```python
from build123d import *

# Parameters (mm, degrees)
F0_W          = 22.5927522406
F0_H          = 49.5025906712
F1_DEPTH      = 10.16
F2_DEPTH      = 3.81
F3_W          = 11.2244246993
F3_H          = 99.0051813424
F4_DEPTH      = 25.4
F6_DEPTH      = 10.16
F7_R          = 2.54
F8_W          = 33.9610797819
F8_H          = 38.1342638284
F8_H_2        = 37.1269418392
F9_DEPTH      = 5.842
F10_R         = 2.54
F11_W         = 99.0051813424
F11_H         = 67.9221570026
F12_DEPTH     = 10.414
F13_W         = 38.620619569
F13_H         = 17.018
F13_W_2       = 37.6479080878
F14_DEPTH     = 3.302
F15_T1_DEPTH  = 88.9685276568
F15_T6_DEPTH  = 27.94
F15_T11_DEPTH = 27.94
F16_W         = 1.1473407503
F16_H         = 14.478
F17_DEPTH     = 3.302
F18_W         = 19.139082171
F18_H         = 29.1566260799
F18_W_2       = 6.5123029053
F18_H_2       = 0.8140355349
F18_W_3       = 18.2694643736
F18_W_4       = 7.5298482552
F18_W_5       = 18.2365168585
F18_W_6       = 7.1228295565
F18_W_7       = 18.1018151343
F18_W_8       = 7.1228314191
F19_DEPTH     = 0.254
F20_DEPTH     = 1.524


# Not quite as in the source:
# - a fillet or chamfer that OpenCascade refuses, or shapes differently, is made with other operations: its cross-section is extruded or revolved along the edge and cut away or added
# - a feature names something its author has since deleted; it is built from what else it names


with BuildPart() as f1:
    # F0 (on Top) → F1 (new body)
    with BuildSketch(Plane.XY):
        with BuildLine():
            Line((-35.3594812499, 51.6611337662), (-36.6952344775, 51.6611337662))
            Line((-36.6952344775, 51.6611337662), (-36.6952344775, 50.3253805386))
            ThreePointArc((-36.6952344775, 50.3253805386), (-36.1400711383, 51.105970427), (-35.3594812499, 51.6611337662))
        make_face()
        with BuildLine():
            ThreePointArc((-32.8504798068, 51.6611337662), (-34.1049805284, 51.9489325583), (-35.3594812499, 51.6611337662))
            Line((-35.3594812499, 51.6611337662), (-32.8504798068, 51.6611337662))
        make_face()
        with BuildLine():
            Line((-32.8504798068, 51.6611337662), (-35.3594812499, 51.6611337662))
            ThreePointArc((-35.3594812499, 51.6611337662), (-36.1400711383, 51.105970427), (-36.6952344775, 50.3253805386))
            Line((-36.6952344775, 50.3253805386), (-36.6952344775, 47.8163790954))
            ThreePointArc((-36.6952344775, 47.8163790954), (-33.4614356183, 46.2656993361), (-31.2269277871, 49.070879817))
            ThreePointArc((-31.2269277871, 49.070879817), (-31.6663634179, 50.5993869876), (-32.8504798068, 51.6611337662))
        make_face()
        with BuildLine():
            Line((-36.6952344775, 47.8163790954), (-36.6952344775, 50.3253805386))
            ThreePointArc((-36.6952344775, 50.3253805386), (-36.9830332696, 49.070879817), (-36.6952344775, 47.8163790954))
        make_face()
        with BuildLine():
            Line((-14.1024822369, 51.6611337662), (-32.8504798068, 51.6611337662))
            ThreePointArc((-32.8504798068, 51.6611337662), (-31.6663634179, 50.5993869876), (-31.2269277871, 49.070879817))
            ThreePointArc((-31.2269277871, 49.070879817), (-33.4614356183, 46.2656993361), (-36.6952344775, 47.8163790954))
            Line((-36.6952344775, 47.8163790954), (-36.6952344775, 2.158543095))
            Line((-36.6952344775, 2.158543095), (-14.1024822369, 2.158543095))
            Line((-14.1024822369, 2.158543095), (-14.1024822369, 51.6611337662))
        make_face()
        with Locations((-2.8061061166, 26.9098384306)):
            Rectangle(F0_W, F0_H)
        with BuildLine():
            Line((-14.1024822369, 2.158543095), (-36.6952344775, 2.158543095))
            Line((-36.6952344775, 2.158543095), (-36.6952344775, -43.4992929054))
            ThreePointArc((-36.6952344775, -43.4992929054), (-33.4614356183, -41.9486131461), (-31.2269277871, -44.753793627))
            ThreePointArc((-31.2269277871, -44.753793627), (-31.6663634179, -46.2823007976), (-32.8504798068, -47.3440475762))
            Line((-32.8504798068, -47.3440475762), (-14.1024822369, -47.3440475762))
            Line((-14.1024822369, -47.3440475762), (-14.1024822369, 2.158543095))
        make_face()
        with Locations((-2.8061061166, -22.5927522406)):
            Rectangle(F0_W, F0_H)
        with BuildLine():
            ThreePointArc((-31.2269277871, -44.753793627), (-33.4614356183, -41.9486131461), (-36.6952344775, -43.4992929054))
            Line((-36.6952344775, -43.4992929054), (-36.6952344775, -46.0082943486))
            ThreePointArc((-36.6952344775, -46.0082943486), (-36.1400711383, -46.788884237), (-35.3594812499, -47.3440475762))
            Line((-35.3594812499, -47.3440475762), (-32.8504798068, -47.3440475762))
            ThreePointArc((-32.8504798068, -47.3440475762), (-31.6663634179, -46.2823007976), (-31.2269277871, -44.753793627))
        make_face()
        with BuildLine():
            Line((-36.6952344775, -46.0082943486), (-36.6952344775, -43.4992929054))
            ThreePointArc((-36.6952344775, -43.4992929054), (-36.9830332696, -44.753793627), (-36.6952344775, -46.0082943486))
        make_face()
        with BuildLine():
            ThreePointArc((-35.3594812499, -47.3440475762), (-36.1400711383, -46.788884237), (-36.6952344775, -46.0082943486))
            Line((-36.6952344775, -46.0082943486), (-36.6952344775, -47.3440475762))
            Line((-36.6952344775, -47.3440475762), (-35.3594812499, -47.3440475762))
        make_face()
        with BuildLine():
            ThreePointArc((-35.3594812499, -47.3440475762), (-34.1049805284, -47.6318463683), (-32.8504798068, -47.3440475762))
            Line((-32.8504798068, -47.3440475762), (-35.3594812499, -47.3440475762))
        make_face()
    extrude(amount=F1_DEPTH)

    # F0 (on Top) → F2 (join)
    with BuildSketch(Plane.XY):
        with BuildLine():
            Line((-32.8504798068, 51.6611337662), (-35.3594812499, 51.6611337662))
            ThreePointArc((-35.3594812499, 51.6611337662), (-36.1400711383, 51.105970427), (-36.6952344775, 50.3253805386))
            Line((-36.6952344775, 50.3253805386), (-36.6952344775, 47.8163790954))
            ThreePointArc((-36.6952344775, 47.8163790954), (-33.4614356183, 46.2656993361), (-31.2269277871, 49.070879817))
            ThreePointArc((-31.2269277871, 49.070879817), (-31.6663634179, 50.5993869876), (-32.8504798068, 51.6611337662))
        make_face()
        with BuildLine():
            ThreePointArc((-31.2269277871, -44.753793627), (-33.4614356183, -41.9486131461), (-36.6952344775, -43.4992929054))
            Line((-36.6952344775, -43.4992929054), (-36.6952344775, -46.0082943486))
            ThreePointArc((-36.6952344775, -46.0082943486), (-36.1400711383, -46.788884237), (-35.3594812499, -47.3440475762))
            Line((-35.3594812499, -47.3440475762), (-32.8504798068, -47.3440475762))
            ThreePointArc((-32.8504798068, -47.3440475762), (-31.6663634179, -46.2823007976), (-31.2269277871, -44.753793627))
        make_face()
    extrude(amount=-F2_DEPTH)

    # F3 (on face) → F4 (join)
    with BuildSketch(Plane.XY.offset(10.16)):
        with Locations((2.878057654, 2.158543095)):
            Rectangle(F3_W, F3_H)
    extrude(amount=F4_DEPTH)

    # F5 (on face) → F6 (join)
    with BuildSketch(Plane.XY.offset(10.16)):
        Polygon((-2.7341546956, 40.4367111623), (-2.7341546956, 51.6611337662), (-32.8504798068, 51.6611337662), (-35.3594812499, 51.6611337662), (-36.6952344775, 51.6611337662), (-36.6952344775, 50.3253805386), (-36.6952344775, 47.8163790954), (-36.6952344775, 40.4367111623), align=None)
        Polygon((-2.7341546956, -47.3440475762), (-2.7341546956, -35.8318164945), (-36.6952344775, -35.8318164945), (-36.6952344775, -43.4992929054), (-36.6952344775, -46.0082943486), (-36.6952344775, -47.3440475762), (-35.3594812499, -47.3440475762), (-32.8504798068, -47.3440475762), align=None)
    extrude(amount=F6_DEPTH)

    # F7
    f7_edges = [f1.edges().sort_by_distance(p)[0] for p in [
        (-2.734155, 2.158543, 35.56),
        (-19.714695, -35.831816, 20.32),
        (-19.714695, -47.344048, 20.32),
        (-19.714695, 51.661134, 20.32),
        (-19.714695, 40.436711, 20.32),
    ]]
    fillet(f7_edges, radius=F7_R)

    # F8 (on face) → F9 (join)
    with BuildSketch(Plane.XY.offset(10.16)):
        with Locations((-19.7146945866, 21.3695792481)):
            Rectangle(F8_W, F8_H)
        with Locations((-19.7146945866, -17.2683455748)):
            Rectangle(F8_W, F8_H_2)
    extrude(amount=F9_DEPTH)

    # F10
    f10_edges = [f1.edges().sort_by_distance(p)[0] for p in [
        (-19.714695, 1.295125, 16.002),
        (-19.714695, 2.302447, 16.002),
        (-36.695234, -17.268346, 16.002),
        (-36.695234, 21.369579, 16.002),
    ]]
    fillet(f10_edges, radius=F10_R)

    # F11 (on face) → F12 (join)
    with BuildSketch(Plane.YZ.offset(8.4902700037)):
        with Locations((2.158543095, 30.0757006044)):
            Rectangle(F11_W, F11_H)
    extrude(amount=-F12_DEPTH)

    # F13 (on face) → F14 (join)
    with BuildSketch(Plane(origin=(-2.7341546956, 0, 0), x_dir=(0, -1, 0), z_dir=(-1, 0, 0))):
        with Locations((-21.1264013778, 24.511)):
            Rectangle(F13_W, F13_H)
        with Locations((17.0078624506, 24.511)):
            Rectangle(F13_W_2, F13_H)
    extrude(amount=F14_DEPTH)

    # F15: fillet of radius 2.54 on 3 edges, made by hand

    # F15_s2 → F15_t1 (cut)
    with BuildSketch(Plane.XZ.offset(-46.7867111623)):
        with BuildLine():
            ThreePointArc((-6.0361546956, 30.48), (-5.2922059199, 32.2760512242), (-3.4961546956, 33.02))
            Line((-3.4961546956, 33.02), (-6.0361546956, 33.02))
            Line((-6.0361546956, 33.02), (-6.0361546956, 30.48))
        make_face()
    extrude(amount=F15_T1_DEPTH, mode=Mode.SUBTRACT)


with BuildPart() as f15_tool4:
    # F15_s5 → F15_t6 (new body)
    with BuildSketch(Plane.XY.offset(39.37)):
        with BuildLine():
            ThreePointArc((-6.0361546956, 37.8967111623), (-5.2922059199, 39.6927623865), (-3.4961546956, 40.4367111623))
            Line((-3.4961546956, 40.4367111623), (-6.0361546956, 40.4367111623))
            Line((-6.0361546956, 40.4367111623), (-6.0361546956, 37.8967111623))
        make_face()
    extrude(amount=-F15_T6_DEPTH)

    split(bisect_by=Plane.XY.offset(16.002), keep=Keep.TOP)


with BuildPart() as f1_1:
    add(f1.part)

    # F15_t3: cut F15_tool4
    add(f15_tool4.part, mode=Mode.SUBTRACT)


with BuildPart() as f15_tool9:
    # F15_s10 → F15_t11 (new body)
    with BuildSketch(Plane.XY.offset(11.43)):
        with BuildLine():
            ThreePointArc((-6.0361546956, -33.2918164945), (-5.2922059199, -35.0878677187), (-3.4961546956, -35.8318164945))
            Line((-3.4961546956, -35.8318164945), (-6.0361546956, -35.8318164945))
            Line((-6.0361546956, -35.8318164945), (-6.0361546956, -33.2918164945))
        make_face()
    extrude(amount=F15_T11_DEPTH)

    split(bisect_by=Plane.XY.offset(16.002), keep=Keep.TOP)


with BuildPart() as f1_2:
    add(f1_1.part)

    # F15_t8: cut F15_tool9
    add(f15_tool9.part, mode=Mode.SUBTRACT)

    # F16 (on face) → F17 (cut)
    with BuildSketch(Plane(origin=(-6.0361546956, 0, 0), x_dir=(0, -1, 0), z_dir=(-1, 0, 0))):
        with Locations((-1.7287769588, 23.241)):
            Rectangle(F16_W, F16_H)
    extrude(amount=-F17_DEPTH, mode=Mode.SUBTRACT)

    # F18 (on face) → F19 (join)
    with BuildSketch(Plane(origin=(-1.9237299963, 0, 0), x_dir=(0, -1, 0), z_dir=(-1, 0, 0))):
        with Locations((-30.8671663515, 49.4584660657)):
            Rectangle(F18_W, F18_H)
        with Locations((-30.3225759417, 61.080571264)):
            Rectangle(F18_W_2, F18_H_2, mode=Mode.SUBTRACT)
        with Locations((-11.2932752818, 49.4584660657)):
            Rectangle(F18_W_3, F18_H)
        with Locations((-11.4979553036, 61.080571264)):
            Rectangle(F18_W_4, F18_H_2, mode=Mode.SUBTRACT)
        with Locations((7.7183801332, 49.4584660657)):
            Rectangle(F18_W_5, F18_H)
        with Locations((7.9371919855, 61.080571264)):
            Rectangle(F18_W_6, F18_H_2, mode=Mode.SUBTRACT)
        with Locations((26.7809126526, 49.4584660657)):
            Rectangle(F18_W_7, F18_H)
        with Locations((27.0670773461, 61.080571264)):
            Rectangle(F18_W_8, F18_H_2, mode=Mode.SUBTRACT)
    extrude(amount=F19_DEPTH)

    # F18 (on face) → F20 (join)
    with BuildSketch(Plane(origin=(-1.9237299963, 0, 0), x_dir=(0, -1, 0), z_dir=(-1, 0, 0))):
        with Locations((27.0670773461, 61.080571264)):
            Rectangle(F18_W_8, F18_H_2)
        with Locations((7.9371919855, 61.080571264)):
            Rectangle(F18_W_6, F18_H_2)
        with Locations((-11.4979553036, 61.080571264)):
            Rectangle(F18_W_4, F18_H_2)
        with Locations((-30.3225759417, 61.080571264)):
            Rectangle(F18_W_2, F18_H_2)
    extrude(amount=F20_DEPTH)


solid = f1_2.part
```
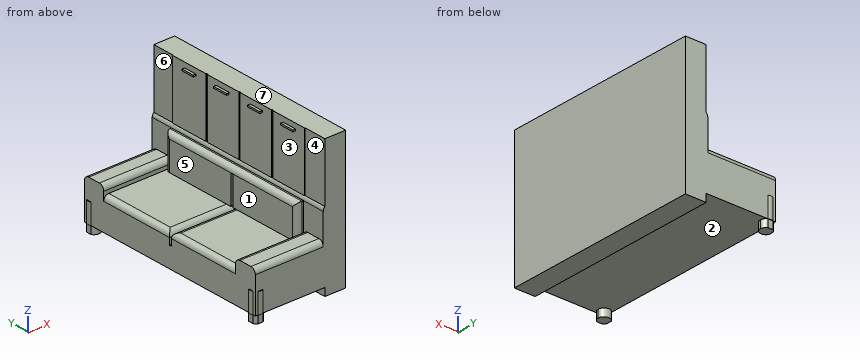
The model under review builds one solid part; all positions refer to its coordinate system, in mm. Face numbers are marked on the shaded views. A direction names the side the tool comes from. Round coordinates to 2 decimals unless told otherwise and drop trailing zeros. Order: outer loops, then holes, each group sorted by start corner. A loop starts at its lowest first (then second) coordinate and runs counter-clockwise, first axis right, second up. Notation, with made-up numbers: (68, -34) -> (82, -34) arc R23 ccw to (82, -22) -> close; hole circle Ø1 at (77.5, -27.5). An arc over 180 degrees is marked (long way). One line per item, written item: value. Start each with the question number.
Q1. Take a section at C-C (z = 22.5). Write out the cut boundary in (x, y).
Q2. Take a section at D-D (y = 35.5). Write out the cut boundary in (x, z), and give its area (3 significant figures).
Q3. Clearance check with flat-ended pins moving along their axes: pin 1 Ø8 at (x, y) = (-29, -12) entering from -Z; pin 2 Ø12 at (x, y) = (-29.5, 18.5) entering from +Z; pin 3 Ø2 at (y, z) = (49.5, -2) entering from -X. State where each tip first meets the part, or that it passes through.
Q4. Mouldability with a two-part tool opening along Z and no side actions: class the marked faces 1, 2 and 3 as released by +Z, released by -Z, zero draft, split by the parting line, or undercut.
Q5. Take a section at A-A (y = 12.5). Write out the cut boundary in (x, z).
Q6. Take a section at B-B (x = -26.5). Write out the cut boundary in (y, z), and give its area (3 significant figures).
Q7. Wall thickness on line 1 (X direction, y = 45, z = 42); line 2 (Z direction, x = -12.5, y = 19.5); line 3 (X direction, y = -7, z = 11.5): over which ranges is each line inside the solid? List them lowest first.
Q8. Machinability: for the marked faces 4, 5, 6 and 7, which of the approach directions +Z, -Z, +X, -X, +Y, -Y give a long, thin tool a straight path to every point of the face, cutting with its end or side? Answer none if there is none.
Reported:
1. outline: (-6.04, -33.29) arc R2.54 ccw to (-3.5, -35.83) -> (-2.73, -35.83) -> (-2.73, -47.34) -> (8.49, -47.34) -> (8.49, 51.66) -> (-2.73, 51.66) -> (-2.73, 40.44) -> (-3.5, 40.44) arc R2.54 ccw to (-6.04, 37.9) -> (-6.04, 2.3) -> (-2.73, 2.3) -> (-2.73, 1.16) -> (-6.04, 1.16) -> close
2. outline: (-36.7, 0) -> (-1.92, 0) -> (-1.92, -3.89) -> (8.49, -3.89) -> (8.49, 64.04) -> (-2.18, 64.04) -> (-2.18, 34.88) -> (-1.92, 34.88) arc R2.54 ccw to (-2.73, 33.02) -> (-3.5, 33.02) arc R2.54 ccw to (-6.04, 30.48) -> (-6.04, 16) -> (-34.16, 16) arc R2.54 ccw to (-36.7, 13.46) -> close
2. area: 1,340 mm2
3. pin 1: stops at z = 0
3. pin 2: stops at z = 16
3. pin 3: stops at x = -36.7
4. face 1: zero draft
4. face 2: released by -Z
4. face 3: undercut
5. outline: (-36.7, 0) -> (-1.92, 0) -> (-1.92, -3.89) -> (8.49, -3.89) -> (8.49, 64.04) -> (-2.18, 64.04) -> (-2.18, 61.49) -> (-3.45, 61.49) -> (-3.45, 60.67) -> (-2.18, 60.67) -> (-2.18, 34.88) -> (-1.92, 34.88) arc R2.54 ccw to (-2.73, 33.02) -> (-3.5, 33.02) arc R2.54 ccw to (-6.04, 30.48) -> (-6.04, 16) -> (-34.16, 16) arc R2.54 ccw to (-36.7, 13.46) -> close
6. outline: (-47.34, 0) -> (51.66, 0) -> (51.66, 17.78) arc R2.54 ccw to (49.12, 20.32) -> (42.98, 20.32) arc R2.54 ccw to (40.44, 17.78) -> (40.44, 16) -> (4.84, 16) arc R2.54 ccw to (2.3, 13.46) -> (2.3, 10.16) -> (1.3, 10.16) -> (1.3, 13.46) arc R2.54 ccw to (-1.24, 16) -> (-35.83, 16) -> (-35.83, 17.78) arc R2.54 ccw to (-38.37, 20.32) -> (-44.8, 20.32) arc R2.54 ccw to (-47.34, 17.78) -> close
6. area: 1,670 mm2
7. line 1: x = -1.92 to 8.49
7. line 2: z = 0 to 16
7. line 3: x = -36.7 to 8.49
8. face 4: +Z, -X, -Y
8. face 5: +Z, -X
8. face 6: +Z, -X, +Y
8. face 7: +Z, +X, -X, +Y, -Y
